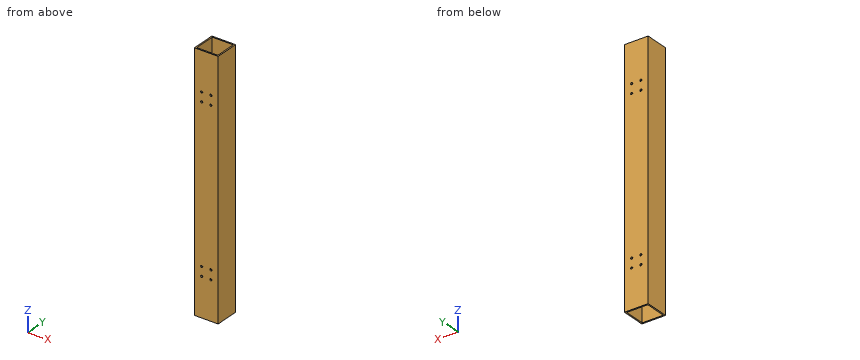
from build123d import *

# Parameters (mm, degrees)
SKETCH1_W               = 34.925
SKETCH1_H               = 34.925
SKETCH1_W_2             = 30.9626
SKETCH1_H_2             = 30.9626
BOSS_EXTRUDE1_DEPTH     = 182.5625
CUT_EXTRUDE1_DEPTH      = 185.22525402
CUT_EXTRUDE1_DEPTH_BACK = 185.22525402
SKETCH2_R               = 1.56250005


with BuildPart() as part:
    # Sketch1 → Boss-Extrude1 (new, symmetric)
    with BuildSketch(Plane.XY):
        Rectangle(SKETCH1_W, SKETCH1_H)
        Rectangle(SKETCH1_W_2, SKETCH1_H_2, mode=Mode.SUBTRACT)
    extrude(amount=BOSS_EXTRUDE1_DEPTH, both=True)

    # Sketch2 → Cut-Extrude1 (cut, two sides: drawn at the far end of the back side and taken through both)
    with BuildSketch(Plane(origin=(0, 0, 0), x_dir=(1, 0, 0), z_dir=(0, 1, 0)).offset(-CUT_EXTRUDE1_DEPTH_BACK)):
        with Locations(Location((-6.717514421, 125.780014421, 0), (0, 0, 270))):
            Circle(SKETCH2_R)
        with Locations(Location((6.717514421, 125.780014421, 0), (0, 0, 270))):
            Circle(SKETCH2_R)
        with Locations(Location((6.717514421, 112.344985579, 0), (0, 0, 270))):
            Circle(SKETCH2_R)
        with Locations(Location((-6.717514421, 112.344985579, 0), (0, 0, 270))):
            Circle(SKETCH2_R)
        with Locations(Location((-6.717514421, -112.344985579, 0), (0, 0, 270))):
            Circle(SKETCH2_R)
        with Locations(Location((6.717514421, -112.344985579, 0), (0, 0, 270))):
            Circle(SKETCH2_R)
        with Locations(Location((6.717514421, -125.780014421, 0), (0, 0, 270))):
            Circle(SKETCH2_R)
        with Locations(Location((-6.717514421, -125.780014421, 0), (0, 0, 270))):
            Circle(SKETCH2_R)
    extrude(amount=CUT_EXTRUDE1_DEPTH + CUT_EXTRUDE1_DEPTH_BACK, mode=Mode.SUBTRACT)


solid = part.part
Could you check a few things on this model? Use its own coordinates, in mm. Round coordinates to 2 decimals unless told otherwise and drop trailing zeros. Loops run counter-clockwise (first coordinate to the right, second up) from the corner with the lowest first, then second, coordinate; pieces in that order, holes last. Notation, with made-up numbers: (-12.5, 2.25) -> (-3.5, 2.25) arc R21 ccw to (-3.5, 37.25) -> close; hole circle Ø8 at (-32.5, 15.5). An arc over 180 degrees is marked (long way). Use CSV: the item, a comma, the result in double quotes.
(1) Suppose I cut it at C-C on z = 33. Write out the boundary of the cut face in (x, y).
Return value:
outline,"(-17.46, -17.46) -> (17.46, -17.46) -> (17.46, 17.46) -> (-17.46, 17.46) -> close; hole (-15.48, -15.48) -> (15.48, -15.48) -> (15.48, 15.48) -> (-15.48, 15.48) -> close"
(2) If I drill on probe 1 along Y at (x, z) = (-13.5, -112), over which ranges is the centre line in solid material (lowest first)? Write a range as [from, to].
Return value:
probe 1,"y = [-17.46, -15.48], [15.48, 17.46]"
(3) Suppose I cut it at A-A on y = -8. Write out the boundary of the cut face in (x, z), plus the area to 3 significant figures.
Return value:
outline,"(-17.46, -182.56) -> (-15.48, -182.56) -> (-15.48, 182.56) -> (-17.46, 182.56) -> close; (15.48, -182.56) -> (17.46, -182.56) -> (17.46, 182.56) -> (15.48, 182.56) -> close"
area,"1,450 mm²"
(4) Will this pin go through, and if not, where does the flat tip stop? pin 1 Ø3.5 at (x, z) = (6.72, -125.78) entering from +Y.
Return value:
pin 1,"stops at y = 17.46"
